Answer from the drawing. Dimensions are ordinates in mm from the lowest x, y and z of the part. A direction names the side the tool comes from. Give positions to 0.01 mm unless a question says otherwise; leave off trailing zeros. Loops run counter-clockwise (first coordinate to the right, second up) from the corner with the lowest first, then second, coordinate; pieces in that order, holes last.
(1) Straight lines are drawn through the part: probe 1 along X at (y, z) = (13, 39) (1 decimal); probe 2 along Y at (x, z) = (20, 37.75); probe 3 along Z at (x, y) = (27, 18). For each, find the intervals that lie inside material, in ascending order.
(2) Find section D-D, the plane y = 35.05. Write down the section's boundary in (x, z).
(3) Find section A-A, the plane y = 20. Write down the section's boundary in (x, z).
(4) Each of these flat-tipped pins is pushed along its axis until it touches: P1, Ø10, axis at x = 15.5, y = 21, coming from the +Z side; P2, Ø4, axis at y = 5.5, z = 22.5, coming from the +X side; P3, Ø1.5, axis at x = 20, y = 35.05, coming from the +Z side; P4, Ø1.5, axis at x = 31.5, z = 19, coming from the -Y side (1 decimal). Where does it stop, or does it pass through?
(5) Find section C-C, the plane z = 18. Write down the section's boundary in (x, y).
(6) Determine the mould class of the marked faces 1, 2 and 3 for opening direction Y: pulls with the +Y half, pulls with the -Y half, needs draft (parallel to the pull), parting line crosses it, or undercut.
(7) Which of the six approach directions +Z, -Z, +X, -X, +Y, -Y give full straight-line access (tool end or side, diameter ignored) to the marked faces 4 and 5?
(8) Find section B-B, the plane x = 20. Write down the section's boundary in (y, z).
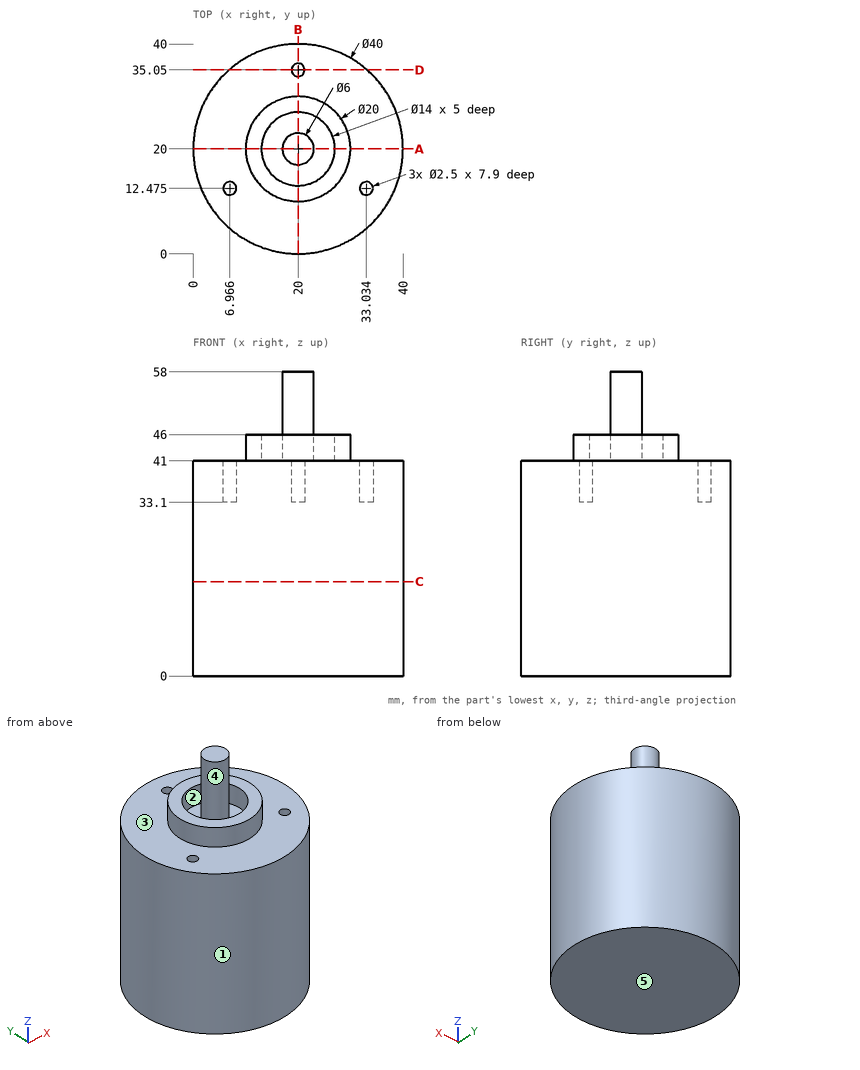
Entries:
1. probe 1: x = 1.3 to 5.8, 8.1 to 31.9, 34.2 to 38.7
1. probe 2: y = 0 to 33.8, 36.3 to 40
1. probe 3: z = 0 to 46
2. outline: (6.83, 0) - (33.17, 0) - (33.17, 41) - (21.25, 41) - (21.25, 33.1) - (18.75, 33.1) - (18.75, 41) - (6.83, 41) - close
3. outline: (0, 0) - (40, 0) - (40, 41) - (30, 41) - (30, 46) - (27, 46) - (27, 41) - (23, 41) - (23, 58) - (17, 58) - (17, 41) - (13, 41) - (13, 46) - (10, 46) - (10, 41) - (0, 41) - close
4. P1: stops at z = 58
4. P2: stops at x = 35.61
4. P3: stops at z = 33.1
4. P4: stops at y = 3.1
5. outline: circle Ø40 at (20, 20)
6. face 1: parting line crosses it
6. face 2: undercut
6. face 3: needs draft
7. face 4: +Z
7. face 5: -Z, +X, -X, +Y, -Y
8. outline: (0, 0) - (40, 0) - (40, 41) - (36.3, 41) - (36.3, 33.1) - (33.8, 33.1) - (33.8, 41) - (30, 41) - (30, 46) - (27, 46) - (27, 41) - (23, 41) - (23, 58) - (17, 58) - (17, 41) - (13, 41) - (13, 46) - (10, 46) - (10, 41) - (0, 41) - close
